```python
from build123d import *

# Parameters (mm, degrees)
RESSALTO_EXTRUS_O1_DEPTH = 6
ESBO_O2_W                = 175
ESBO_O2_H                = 6.1
CORTE_EXTRUS_O1_DEPTH    = 10
ESBO_O3_R                = 5.725
CORTE_EXTRUS_O2_DEPTH    = 10


with BuildPart() as part:
    # Esboço1 → Ressalto-extrusão1 (new body)
    with BuildSketch(Plane.XY):
        Polygon((-67, -97), (-97, -97), (-97, 97), (-67, 97), (-67, 103), (-37, 103), (-37, 97), (43, 97), (43, 103), (73, 103), (73, 97), (97, 97), (97, -97), (73, -97), (73, -103), (43, -103), (43, -97), (-37, -97), (-37, -103), (-67, -103), align=None)
    extrude(amount=RESSALTO_EXTRUS_O1_DEPTH)

    # Esboço2 → Corte-extrusão1 (cut)
    with BuildSketch(Plane.XY.offset(6)):
        with Locations((-9.5, 3.05)):
            Rectangle(ESBO_O2_W, ESBO_O2_H)
        with Locations((-9.5, -87.85)):
            Rectangle(ESBO_O2_W, ESBO_O2_H)
    extrude(amount=-CORTE_EXTRUS_O1_DEPTH, mode=Mode.SUBTRACT)

    # Esboço3 → Corte-extrusão2 (cut)
    with BuildSketch(Plane.XY.offset(6)):
        with Locations((-77, -63)):
            Circle(ESBO_O3_R)
    extrude(amount=-CORTE_EXTRUS_O2_DEPTH, mode=Mode.SUBTRACT)


solid = part.part
```
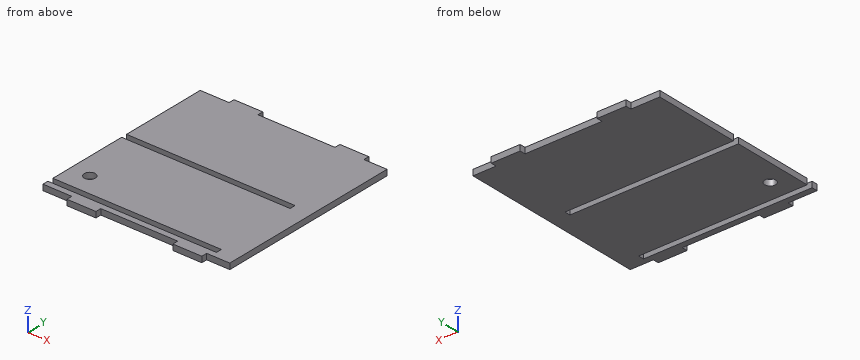
Geometry check sheet. Reference: the model listing, model coordinates, mm. Coordinates: 2 decimals unless noted, no trailing zeros. Write each loop counter-clockwise with the first axis right and the second up, starting at its lowest first coordinate (ties: lowest second). Pieces come first, ordered by that corner, then holes. Notation, with made-up numbers: M 2,64.5 L 8,64.5 A19 ccw 8,78.5 Z; hole C 58.5,-14.5 d10. An arc over 180 degrees is marked long. Use one line per item in the form item = value. Start each with the question number.
1) Section check A-A on x = -77. Enter the section's corners in (y, z) (3 decimals).
2) Thickness scan on probe 1 along Y at (x, z) = (-50, 5.65); probe 2 along Y at (x, z) = (-25.5, 1.3); probe 3 along Y at (x, z) = (-77, 1.6) (3 decimals). Record the ranges inside material, lowest first. Write a range as from..to.
3) Go/stop test with flat-tipped pins: pin 1 Ø3 at (x, z) = (85, 1.5) entering from +Y; pin 2 Ø3 at (y, z) = (-87, 4) entering from -X; pin 3 Ø3 at (y, z) = (100, 2) entering from -X. Record where each tip stops, or that it passes through.
4) Section check B-B on y = -63. Enter the section's corners in (x, z) (3 decimals).
5) Section check C-C on x = 20. Enter the section's corners in (y, z), and give its area (3 significant figures).
Responses:
q1.outline = M -97,0 L -90.9,0 L -90.9,6 L -97,6 Z; M -84.8,0 L -68.725,0 L -68.725,6 L -84.8,6 Z; M -57.275,0 L 0,0 L 0,6 L -57.275,6 Z; M 6.1,0 L 97,0 L 97,6 L 6.1,6 Z
q2.probe_1 = -103..-90.9, -84.8..0, 6.1..103
q2.probe_2 = -97..-90.9, -84.8..0, 6.1..97
q2.probe_3 = -97..-90.9, -84.8..-68.725, -57.275..0, 6.1..97
q3.pin_1 = 97
q3.pin_2 = 78
q3.pin_3 = -67
q4.outline = M -97,0 L -82.725,0 L -82.725,6 L -97,6 Z; M -71.275,0 L 97,0 L 97,6 L -71.275,6 Z
q5.outline = M -97,0 L -90.9,0 L -90.9,6 L -97,6 Z; M -84.8,0 L 0,0 L 0,6 L -84.8,6 Z; M 6.1,0 L 97,0 L 97,6 L 6.1,6 Z
q5.area = 1,090 mm2
